CAD build for the part. Positions are in the model's coordinates, mm. Coordinates: 2 decimals unless noted, no trailing zeros. Write each loop counter-clockwise with the first axis right and the second up, starting at its lowest first coordinate (ties: lowest second). Pieces come first, ordered by that corner, then holes.
```python
from build123d import *

# Parameters (mm, degrees)
SKETCH2_R               = 2.3495
SKETCH2_R_2             = 2.0955
BOSS_EXTRUDE1_DEPTH     = 2.54
SKETCH3_W               = 31.75
SKETCH3_H               = 44.323
BOSS_EXTRUDE2_DEPTH     = 2.54
SKETCH4_R               = 2.413
CUT_EXTRUDE1_DEPTH      = 238.743265275
SKETCH5_R               = 2.413
CUT_EXTRUDE2_DEPTH      = 238.743265275
SKETCH6_R               = 2.413
CUT_EXTRUDE3_DEPTH      = 238.743265275
SKETCH7_R               = 2.413
CUT_EXTRUDE4_DEPTH      = 238.743265275
SKETCH8_W               = 7.994763
SKETCH8_H               = 21.113506736
SKETCH8_W_2             = 21.493659396
SKETCH8_H_2             = 28.960940125
CUT_EXTRUDE5_DEPTH      = 238.743265275
CUT_EXTRUDE6_DEPTH      = 238.743265275
CUT_EXTRUDE6_DEPTH_BACK = 238.743265275
CUT_EXTRUDE7_REACH      = 206.142
SKETCH10_R              = 2.3495
FILLET1_R               = 1.5875


with BuildPart() as part:
    # Sketch2 → Boss-Extrude1 (new body)
    with BuildSketch(Plane(origin=(0, 0, 0), x_dir=(-1, 0, 0), z_dir=(0, 0, 1))):
        Polygon((-2.930050059, 168.708281075), (38.709428475, 168.708281075), (38.709428475, 189.536281075), (143.497061781, 189.536281075), (104.617436481, 110.859781075), (72.867436481, 110.859781075), (72.867436481, 66.536781075), (104.617436481, 66.536781075), (143.497061781, -12.139718925), (38.709428475, -12.139718925), (38.709428475, 8.688281075), (-2.930050059, 8.688281075), align=None)
        with Locations(Location((41.95655448, 160.961281075, 0), (0, 0, 180))):
            Circle(SKETCH2_R, mode=Mode.SUBTRACT)
        with Locations(Location((90.673911143, 180.011281075, 0), (0, 0, 180))):
            Circle(SKETCH2_R, mode=Mode.SUBTRACT)
        with Locations(Location((90.673911143, -2.614718925, 0), (0, 0, 180))):
            Circle(SKETCH2_R, mode=Mode.SUBTRACT)
        with Locations(Location((3.035061781, 117.209781075, 0), (0, 0, 180))):
            Circle(SKETCH2_R, mode=Mode.SUBTRACT)
        with Locations(Location((3.035061781, 60.186781075, 0), (0, 0, 180))):
            Circle(SKETCH2_R, mode=Mode.SUBTRACT)
        with Locations(Location((41.95655448, 16.435281075, 0), (0, 0, 180))):
            Circle(SKETCH2_R_2, mode=Mode.SUBTRACT)
    extrude(amount=BOSS_EXTRUDE1_DEPTH)

    # Sketch3 → Boss-Extrude2 (add)
    with BuildSketch(Plane.XY.offset(2.54)):
        with Locations((-88.742436481, -88.698281075)):
            Rectangle(SKETCH3_W, SKETCH3_H)
    extrude(amount=-BOSS_EXTRUDE2_DEPTH)

    # Sketch4 → Cut-Extrude1 (cut, through all)
    with BuildSketch(Plane.XY.offset(2.54)):
        with Locations((-96.39567787, -68.835481075)):
            Circle(SKETCH4_R)
        with Locations((-84.96567787, -68.835481075)):
            Circle(SKETCH4_R)
        with Locations((-30.343949941, -66.422481075)):
            Circle(SKETCH4_R)
        with Locations((-11.293949941, -66.422481075)):
            Circle(SKETCH4_R)
        with Locations(Location((-11.293949941, -110.974081075, 0), (0, 0, 180))):
            Circle(SKETCH4_R)
        with Locations(Location((-30.343949941, -110.974081075, 0), (0, 0, 180))):
            Circle(SKETCH4_R)
        with Locations(Location((-84.96567787, -108.561081075, 0), (0, 0, 180))):
            Circle(SKETCH4_R)
        with Locations(Location((-96.39567787, -108.561081075, 0), (0, 0, 180))):
            Circle(SKETCH4_R)
    extrude(amount=-CUT_EXTRUDE1_DEPTH, mode=Mode.SUBTRACT)

    # Sketch5 → Cut-Extrude2 (cut, through all)
    with BuildSketch(Plane.XY.offset(2.54)):
        with Locations((-31.738991634, -58.273080522)):
            Circle(SKETCH5_R)
    extrude(amount=-CUT_EXTRUDE2_DEPTH, mode=Mode.SUBTRACT)

    # Sketch6 → Cut-Extrude3 (cut, through all)
    with BuildSketch(Plane.XY.offset(2.54)):
        with Locations((-32.511395831, -23.991781075)):
            Circle(SKETCH6_R)
    extrude(amount=-CUT_EXTRUDE3_DEPTH, mode=Mode.SUBTRACT)

    # Sketch7 → Cut-Extrude4 (cut, through all)
    with BuildSketch(Plane.XY.offset(2.54)):
        with Locations((-32.140467993, -155.071444629)):
            Circle(SKETCH7_R)
        with Locations((-32.140467993, -120.781444629)):
            Circle(SKETCH7_R)
    extrude(amount=-CUT_EXTRUDE4_DEPTH, mode=Mode.SUBTRACT)

    # Sketch8 → Cut-Extrude5 (cut, through all)
    with BuildSketch(Plane.XY.offset(2.54)):
        with Locations((-36.236046975, 1.868472293)):
            Rectangle(SKETCH8_W, SKETCH8_H)
        with Locations((-29.486598777, -183.188751137)):
            Rectangle(SKETCH8_W_2, SKETCH8_H_2)
    extrude(amount=-CUT_EXTRUDE5_DEPTH, mode=Mode.SUBTRACT)

    # Sketch9 → Cut-Extrude6 (cut, two sides: drawn at the far end of the back side and taken through both)
    with BuildSketch(Plane.XY.offset(2.54).offset(-CUT_EXTRUDE6_DEPTH_BACK)):
        Polygon((-104.617436481, -66.536781075), (-104.617436481, 15.636566552), (-183.179161499, 15.636566552), (-188.262141255, -199.721259961), (-104.617436481, -202.664037714), align=None)
    extrude(amount=CUT_EXTRUDE6_DEPTH + CUT_EXTRUDE6_DEPTH_BACK, mode=Mode.SUBTRACT)

    # Sketch10 → Cut-Extrude7 (cut, up to next)
    with BuildSketch(Plane(origin=(-13.551580143, -6.849856516, 2.54), x_dir=(-0.9999147240311792, 0.01305927508136085, 0), z_dir=(0, 0, 1)), mode=Mode.PRIVATE) as cut_extrude7_sk1:
        with Locations(Location((46.679311403, -8.178590001, 0), (0, 0, 180.748262615))):
            Circle(SKETCH10_R)
    cut_extrude7_tool1 = extrude(cut_extrude7_sk1.sketch, amount=-CUT_EXTRUDE7_REACH, mode=Mode.PRIVATE) & part.part
    # Sketch10 → Cut-Extrude7 (cut, up to next)
    with BuildSketch(Plane(origin=(-13.551580143, -6.849856516, 2.54), x_dir=(-0.9999147240311792, 0.01305927508136085, 0), z_dir=(0, 0, 1)), mode=Mode.PRIVATE) as cut_extrude7_sk2:
        with Locations(Location((44.406688666, 173.16194469, 0), (0, 0, 180.748262615))):
            Circle(SKETCH10_R)
    cut_extrude7_tool2 = extrude(cut_extrude7_sk2.sketch, amount=-CUT_EXTRUDE7_REACH, mode=Mode.PRIVATE) & part.part
    add(cut_extrude7_tool1.solids().sort_by_distance((-60.120104, 1.937634, 2.54))[0], mode=Mode.SUBTRACT)
    add(cut_extrude7_tool2.solids().sort_by_distance((-60.215851, -179.417115, 2.54))[0], mode=Mode.SUBTRACT)

    # Fillet1
    fillet1_edges = [part.edges().sort_by_distance(p)[0] for p in [
        (-40.233428475, -189.536281075, 1.27),
        (-40.233428475, 12.139718925, 1.27),
        (-40.233428475, -8.688281075, 1.27),
        (-40.233428475, -168.708281075, 1.27),
        (-104.617436481, -189.536281075, 1.27),
        (-104.617436481, 12.139718925, 1.27),
        (2.930050059, -168.708281075, 1.27),
        (2.930050059, -8.688281075, 1.27),
    ]]
    fillet(fillet1_edges, radius=FILLET1_R)


solid = part.part
```
Item 1: Saw through at B-B, the plane y = -5. Write the cut outline in (x, z).
Item 2: Saw through at C-C, the plane z = 2. State how many separate pieces and enclosed holes the cut face has, and give its area (3 significant figures).
Item 3: Wall check: line 1 along Y through (x, z) = (-95, 1.85); line 2 along Y through (x, z) = (-86, 1.4); line 3 along Y through (x, z) = (-37, 0.6). Give the ranges that are in metal, low to high.
Item 4: Flat gauge pins, fed straight in: pin 1 Ø6.5 at (x, y) = (-96.4, -108.56) entering from +Z; pin 2 Ø0.8 at (x, z) = (-17, 1.5) entering from -Y; pin 3 Ø1.3 at (x, z) = (-13.5, 1.5) entering from +Y. Where does each tip first touch, or does it go through?
Item 5: Saw through at A-A, the plane x = -22. Write the cut outline in (y, z), and give its area (3 significant figures).
Item 6: Two-plate mould, pull along Y, no slides. Class faces 1 (the flat face through (-52, -87, 0)), 2 (the cylindrical face through (-29.82, -108.62, 1.29)): +Y half, -Y half, draft (parallel to the pull), parting line (faces both ways), or undercut.
Working result:
1. outline: (-104.62, 0) - (-40.23, 0) - (-40.23, 2.54) - (-104.62, 2.54) - close
2. separate pieces: 1
2. enclosed holes: 20
2. area: 19,500 mm2
3. line 1: y = -189.54 to -110.53, -106.59 to -70.8, -66.87 to 12.14
3. line 2: y = -189.54 to -110.74, -106.38 to -71.02, -66.66 to 12.14
3. line 3: y = -168.71 to -8.69
4. pin 1: stops at z = 2.54
4. pin 2: stops at y = -168.71
4. pin 3: stops at y = -8.69
5. outline: (-168.71, 0) - (-8.69, 0) - (-8.69, 2.54) - (-168.71, 2.54) - close
5. area: 406 mm2
6. face 1: draft
6. face 2: undercut
